```python
from build123d import *

# Parameters (mm, degrees)
F1_DEPTH = 3.175
F0_W     = 180.639096
F0_H     = 5.08
F2_DEPTH = 6.35
F3_DEPTH = 3.175
F4_DEPTH = 3.175
F5_DEPTH = 20.32


with BuildPart() as f1:
    # F0 (on Top) → F1 (new body)
    with BuildSketch(Plane.XY):
        Polygon((185.450711, 51.289835), (172.750711, 51.289835), (172.750711, 38.589835), (185.450711, 38.589835), (185.450711, 45.141608), align=None)
        Polygon((172.750711, 64.923577), (-7.888385, 64.923577), (-7.888385, 51.491608), (4.811615, 51.491608), (4.811615, 45.141608), (4.811615, 38.791608), (-7.888385, 38.791608), (-7.888385, 24.283577), (172.750711, 24.283577), (172.750711, 38.589835), (172.750711, 51.289835), align=None)
    extrude(amount=F1_DEPTH)

    # F0 (on Top) → F2 (join)
    with BuildSketch(Plane.XY):
        with Locations((82.431163, 21.743577)):
            Rectangle(F0_W, F0_H)
        with Locations((82.431163, 67.463577)):
            Rectangle(F0_W, F0_H)
    extrude(amount=F2_DEPTH)

    # F0 (on Top) → F3 (join)
    with BuildSketch(Plane.XY):
        Polygon((-7.888385, 95.403577), (-7.888385, 70.003577), (172.750711, 70.003577), (172.451615, 95.446534), (161.021615, 95.446534), (161.021615, 72.725058), (148.321615, 72.725058), (148.321615, 95.446534), (136.891615, 95.446534), (136.891615, 73.213689), (124.191615, 73.213689), (124.191615, 95.446534), (112.761615, 95.446534), (112.761615, 73.213689), (100.061615, 73.213689), (100.061615, 95.446534), (88.631615, 95.446534), (88.631615, 74.190959), (75.931615, 74.190959), (75.931615, 95.202222), (64.501615, 95.202222), (64.501615, 73.458008), (51.801615, 73.458008), (51.801615, 95.446534), (40.371615, 95.446534), (40.371615, 73.458008), (27.671615, 73.458008), (27.671615, 95.202215), (16.241615, 95.202215), (16.241615, 72.96937), (3.541615, 72.96937), (3.541615, 95.403577), align=None)
        Polygon((172.750711, 19.203577), (-7.888385, 19.203577), (-7.888385, -5.6889), (3.541615, -5.6889), (3.541615, 14.589407), (16.241615, 14.589407), (16.241615, -5.933219), (27.671615, -5.933219), (27.671615, 14.345091), (40.371615, 14.345091), (40.371615, -5.6889), (51.801615, -5.6889), (51.801615, 13.612141), (64.501615, 13.612141), (64.501615, -5.6889), (75.931615, -5.6889), (75.931615, 13.612141), (88.631615, 13.612141), (88.631615, -5.6889), (100.061615, -5.6889), (100.061615, 13.367824), (112.761615, 13.367824), (112.761615, -6.177533), (124.191615, -6.177533), (124.191615, 13.367824), (136.891615, 13.367824), (136.891615, -6.421852), (148.321615, -6.421852), (148.321615, 13.123516), (161.021615, 13.123516), (161.021615, -5.933208), (172.451615, -5.933208), align=None)
    extrude(amount=F3_DEPTH)

    # F0 (on Top) → F4 (join)
    with BuildSketch(Plane.XY):
        Polygon((-7.888385, 95.403577), (-7.888385, 70.003577), (172.750711, 70.003577), (172.451615, 95.446534), (161.021615, 95.446534), (161.021615, 72.725058), (148.321615, 72.725058), (148.321615, 95.446534), (136.891615, 95.446534), (136.891615, 73.213689), (124.191615, 73.213689), (124.191615, 95.446534), (112.761615, 95.446534), (112.761615, 73.213689), (100.061615, 73.213689), (100.061615, 95.446534), (88.631615, 95.446534), (88.631615, 74.190959), (75.931615, 74.190959), (75.931615, 95.202222), (64.501615, 95.202222), (64.501615, 73.458008), (51.801615, 73.458008), (51.801615, 95.446534), (40.371615, 95.446534), (40.371615, 73.458008), (27.671615, 73.458008), (27.671615, 95.202215), (16.241615, 95.202215), (16.241615, 72.96937), (3.541615, 72.96937), (3.541615, 95.403577), align=None)
        with Locations((82.431163, 67.463577)):
            Rectangle(F0_W, F0_H)
        Polygon((172.750711, 64.923577), (-7.888385, 64.923577), (-7.888385, 51.491608), (4.811615, 51.491608), (4.811615, 45.141608), (4.811615, 38.791608), (-7.888385, 38.791608), (-7.888385, 24.283577), (172.750711, 24.283577), (172.750711, 38.589835), (172.750711, 51.289835), align=None)
        Polygon((4.811615, 51.491608), (-7.888385, 51.491608), (-7.888385, 38.791608), (4.811615, 38.791608), (4.811615, 45.141608), align=None)
        Polygon((185.450711, 51.289835), (172.750711, 51.289835), (172.750711, 38.589835), (185.450711, 38.589835), (185.450711, 45.141608), align=None)
        with Locations((82.431163, 21.743577)):
            Rectangle(F0_W, F0_H)
        Polygon((172.750711, 19.203577), (-7.888385, 19.203577), (-7.888385, -5.6889), (3.541615, -5.6889), (3.541615, 14.589407), (16.241615, 14.589407), (16.241615, -5.933219), (27.671615, -5.933219), (27.671615, 14.345091), (40.371615, 14.345091), (40.371615, -5.6889), (51.801615, -5.6889), (51.801615, 13.612141), (64.501615, 13.612141), (64.501615, -5.6889), (75.931615, -5.6889), (75.931615, 13.612141), (88.631615, 13.612141), (88.631615, -5.6889), (100.061615, -5.6889), (100.061615, 13.367824), (112.761615, 13.367824), (112.761615, -6.177533), (124.191615, -6.177533), (124.191615, 13.367824), (136.891615, 13.367824), (136.891615, -6.421852), (148.321615, -6.421852), (148.321615, 13.123516), (161.021615, 13.123516), (161.021615, -5.933208), (172.451615, -5.933208), align=None)
    extrude(amount=F4_DEPTH)

    # F0 (on Top) → F5 (cut)
    with BuildSketch(Plane.XY):
        Polygon((4.811615, 51.491608), (-7.888385, 51.491608), (-7.888385, 38.791608), (4.811615, 38.791608), (4.811615, 45.141608), align=None)
    extrude(amount=F5_DEPTH, mode=Mode.SUBTRACT)


solid = f1.part
```
Build history of the part. All positions in model axes, mm. A direction names the side the tool comes from. Round coordinates to 2 decimals unless told otherwise and drop trailing zeros. Write each loop counter-clockwise with the first axis right and the second up, starting at its lowest first coordinate (ties: lowest second). Pieces come first, ordered by that corner, then holes. Notation, with made-up numbers: (-9.5, 49.5) - (10.5, 49.5) arc R21 ccw to (10.5, 58.5) - close; hole circle Ø1 at (55, -29.75). An arc over 180 degrees is marked (long way). Write each question's results on one line, items separated by ' | '. Start each with the question number.
Item 1: Saw through at C-C (y = 88). State how many separate pieces and enclosed holes the cut face has, and give its area (3 significant figures).
Item 2: Saw through at A-A (z = 4.5). Write the cut outline in (x, y).
Item 3: Saw through at D-D (x = 36). Write the cut outline in (y, z) (3 decimals), and give its area (3 significant figures).
Item 4: Drop flat-ended pins along their axis: P1, Ø7.5, axis at x = 85.5, y = 86, coming from the +Z side (3 decimals); P2, Ø3.5, axis at y = 2.5, z = 1, coming from the +X side; P3, Ø1.9, axis at y = 32, z = 2.5, coming from the +X side. Give the stop position or say it passes through.
Item 5: Which spindle directions (+Z, -Z, +X, -X, +Y, -Y) get a long thin tool onto all of the face, cutting with end or side? Do faces 1 (the face through (81, 15, 3.175)), 2 (the face through (81, 72, 3.175)), 3 (the face through (172.751, 63, 2)), 4 (the face through (172.751, 27, 2)), 5 (the face through (66, 45, 0)). Say none if no direction does.
Item 6: Wall check: L1, parallel to Y at x = 18, z = 5.75; L2, parallel to Y at x = 176.5, z = 2; L3, parallel to Z at x = 1, y = 54.5 (3 decimals). Give the ranges that are in metal, low to high. Write a range as [from, to].
Item 7: Mould opens along Y. For faces 6 (the face through (-7.888, 17, 2)), 7 (the face through (87, 45, 3.175)) say: pulls with the +Y half, pulls with the -Y half, needs draft (parallel to the pull), parting line crosses it, or undercut.
Item 8: Saw through at B-B (x = 79.5). Write the cut outline in (y, z) (3 decimals), and give its area (3 significant figures).
Results are:
1) separate pieces: 8 | enclosed holes: 0 | area: 291 mm²
2) outline: (-7.89, 19.2) - (172.75, 19.2) - (172.75, 24.28) - (-7.89, 24.28) - close; (-7.89, 64.92) - (172.75, 64.92) - (172.75, 70) - (-7.89, 70) - close
3) outline: (14.345, 0) - (73.458, 0) - (73.458, 3.175) - (70.004, 3.175) - (70.004, 6.35) - (64.924, 6.35) - (64.924, 3.175) - (24.284, 3.175) - (24.284, 6.35) - (19.204, 6.35) - (19.204, 3.175) - (14.345, 3.175) - close | area: 220 mm²
4) P1: stops at z = 3.175 | P2: stops at x = 172.57 | P3: stops at x = 172.75
5) face 1: +Z, +X, -X, -Y | face 2: +Z, +X, -X, +Y | face 3: +Z, -Z, +X, +Y | face 4: +Z, -Z, +X, -Y | face 5: -Z, +X, -X, +Y, -Y
6) L1: y = [19.2, 24.28], [64.92, 70] | L2: y = [38.59, 51.29] | L3: z = [0, 3.175]
7) face 6: needs draft | face 7: undercut
8) outline: (13.612, 0) - (74.191, 0) - (74.191, 3.175) - (70.004, 3.175) - (70.004, 6.35) - (64.924, 6.35) - (64.924, 3.175) - (24.284, 3.175) - (24.284, 6.35) - (19.204, 6.35) - (19.204, 3.175) - (13.612, 3.175) - close | area: 225 mm²
